The listing builds one solid part. Answer for the finished solid, in the listing's coordinates (mm). A direction names the side the tool comes from. Give positions to 0.01 mm unless a question says otherwise; leave off trailing zeros. Loops run counter-clockwise (first coordinate to the right, second up) from the corner with the lowest first, then second, coordinate; pieces in that order, holes last. Notation, with made-up numbers: (56.25, -18.75) - (73.25, -18.75) arc R17 cw to (73.25, 7.25) - close; hole circle Ø2 at (7.5, -9). An arc over 180 degrees is marked (long way). Answer in a Markdown table with one row per item. Add a question column.
```python
from build123d import *

# Parameters (mm, degrees)
PAD_DEPTH       = 11
SKETCH001_R     = 3.25
POCKET_DEPTH    = 6
SKETCH002_R     = 3.25
POCKET001_DEPTH = 6
FILLET_R        = 1


with BuildPart() as part:
    # Sketch → Pad (new body, symmetric)
    with BuildSketch(Plane.YZ):
        Polygon((-60, 0), (0, 0), (42.4264068712, 42.4264068712), (38.1837661841, 46.6690475583), (13.7781745931, 22.2634559673), (-25.4852813742, 6), (-60, 6), align=None)
        Polygon((8.1213203436, 16.6066017178), (-17.4852813742, 6), (-2.4852813742, 6), align=None, mode=Mode.SUBTRACT)
    extrude(amount=PAD_DEPTH, both=True)

    # Sketch001 (on Face6 of Pad) → Pocket (cut)
    with BuildSketch(Plane(origin=(0, 0, 6), x_dir=(0, -1, 0), z_dir=(0, 0, 1))):
        with Locations((50, 0)):
            Circle(SKETCH001_R)
    extrude(amount=-POCKET_DEPTH, mode=Mode.SUBTRACT)

    # Sketch002 (on Face9 of Pocket) → Pocket001 (cut)
    with BuildSketch(Plane(origin=(0, -4.2426406871, 4.2426406871), x_dir=(0, -0.7071067812, -0.7071067812), z_dir=(0, -0.7071067812, 0.7071067812))):
        with Locations((-50, 0)):
            Circle(SKETCH002_R)
    extrude(amount=-POCKET001_DEPTH, mode=Mode.SUBTRACT)

    # Fillet
    fillet_edges = [part.edges().sort_by_distance(p)[0] for p in [
        (0, 0, 0),
        (0, -60, 0),
        (0, -60, 6),
        (0, 38.183766, 46.669048),
        (0, 42.426407, 42.426407),
    ]]
    fillet(fillet_edges, radius=FILLET_R)


solid = part.part
```
(1) Find the intervals of material crossed by line 1 along X through (y, z) = (-50, 2); line 2 along Z through (x, y) = (4.75, -47.5); line 3 along Y through (x, z) = (-6.5, 13.5), in increasing order. Write a range as [from, to].
(2) Given pin 1 Ø7.5 at (x, y) = (1, -9.5) entering from +Z; pin 2 Ø11 at (x, y) = (-2.5, -50.5) entering from +Z; pin 3 Ø12 at (x, y) = (-3.5, 5) entering from +Z, each flat-ended and moving along its own axis, determine where each tip first touches the part or whether it passes through.
(3) A cutting plane is placed at D-D on y = -4. Determine the outline of the cut face in (x, z), plus the area to 3 significant figures.
(4) A tool of negligible diameter and unlimited length cuts with its end or side. For faces 5 (the face through (0, -42, 6)), 6 (the face through (-11, -5, 13)), 7 (the face through (0.15, -4.5, 11.38)), from which of +Z, -Z, +X, -X, +Y, -Y can it reach the whole face along a straight path? Write none if from no direction.
(5) A cutting plane is placed at A-A on x = -8.25. Determine the outline of the cut face in (y, z).
(6) The mould has two halves that part along Z. Classify faces 1 (the face through (0.154, 25.793, 34.279)), 2 (the face through (0.154, 2.744, 11.229)), 3 (the face through (-1.245, -53.002, 3.042)), 4 (the face through (0, 21, 21)): pulls with the +Z half, pulls with the -Z half, needs draft (parallel to the pull), parting line crosses it, or undercut.
(7) A cutting plane is placed at B-B on y = -50. Determine the outline of the cut face in (x, z), plus the area to 3 significant figures.
(8) A cutting plane is placed at C-C on x = 0. Determine the outline of the cut face in (y, z), plus the area to 3 significant figures.
Evaluation:
| question | item | result |
|---|---|---|
| 1 | line 1 | x = [-11, -3.25], [3.25, 11] |
| 1 | line 2 | z = [0, 6] |
| 1 | line 3 | y = [-7.38, 0.62], [5.01, 13.5] |
| 2 | pin 1 | stops at z = 14.17 |
| 2 | pin 2 | stops at z = 6 |
| 2 | pin 3 | stops at z = 21.11 |
| 3 | outline | (-11, 0) - (11, 0) - (11, 6) - (-11, 6) - close; (-11, 11.59) - (11, 11.59) - (11, 14.9) - (-11, 14.9) - close |
| 3 | area | 205 mm² |
| 4 | face 5 | +Z, +X, -X, -Y |
| 4 | face 6 | +Z, -Z, -X, +Y, -Y |
| 4 | face 7 | +X, -X |
| 5 | outline | (-60, 1) arc R1 ccw to (-59, 0) - (-0.41, 0) arc R1 ccw to (0.29, 0.29) - (41.72, 41.72) arc R1 ccw to (41.72, 43.13) - (38.89, 45.96) arc R1 ccw to (37.48, 45.96) - (13.78, 22.26) - (-25.49, 6) - (-59, 6) arc R1 ccw to (-60, 5) - close; hole (-17.49, 6) - (-2.49, 6) - (8.12, 16.61) - close |
| 6 | face 1 | pulls with the +Z half |
| 6 | face 2 | undercut |
| 6 | face 3 | needs draft |
| 6 | face 4 | pulls with the -Z half |
| 7 | outline | (-11, 0) - (-3.25, 0) - (-3.25, 6) - (-11, 6) - close; (3.25, 0) - (11, 0) - (11, 6) - (3.25, 6) - close |
| 7 | area | 93.0 mm² |
| 8 | outline | (-60, 1) arc R1 ccw to (-59, 0) - (-53.25, 0) - (-53.25, 6) - (-59, 6) arc R1 ccw to (-60, 5) - close; (-46.75, 0) - (-0.41, 0) arc R1 ccw to (0.29, 0.29) - (33.06, 33.06) - (28.81, 37.3) - (13.78, 22.26) - (-25.49, 6) - (-46.75, 6) - close; (33.41, 41.9) - (37.65, 37.65) - (41.72, 41.72) arc R1 ccw to (41.72, 43.13) - (38.89, 45.96) arc R1 ccw to (37.48, 45.96) - close; hole (-17.49, 6) - (-2.49, 6) - (8.12, 16.61) - close |
| 8 | area | 734 mm² |
